The listing builds one solid part. Answer for the finished solid, in the listing's coordinates (mm). Coordinates: 2 decimals unless noted, no trailing zeros. Write each loop counter-clockwise with the first axis right and the second up, starting at its lowest first coordinate (ties: lowest second). Pieces come first, ordered by that corner, then holes. Notation, with made-up numbers: M 88.5,42 L 103.5,42 A22 ccw 103.5,54 Z; hole C -38,84 d9. An arc over 180 degrees is marked long. Answer as CSV lines item,"result". Start each with the question number.
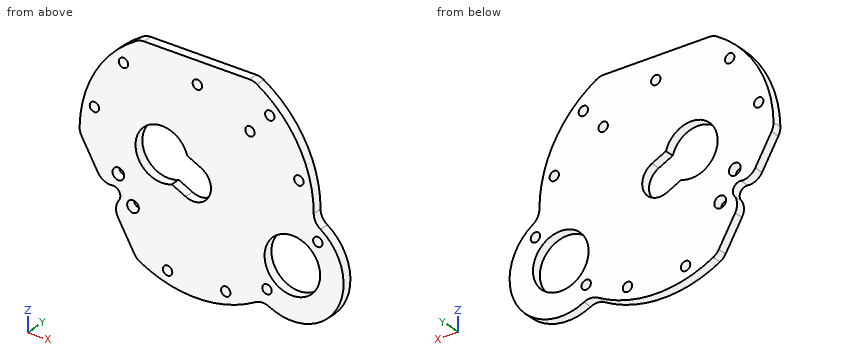
```python
from build123d import *

# Parameters (mm, degrees)
SKETCH2_R           = 9.5
SKETCH2_R_2         = 1.599999999
BOSS_EXTRUDE1_DEPTH = 3.175
FILLET1_R           = 5
CUT_EXTRUDE1_REACH  = 5.175
SKETCH3_R           = 2
FILLET2_R           = 5


with BuildPart() as part:
    # Sketch2 → Boss-Extrude1 (new body)
    with BuildSketch(Plane(origin=(0, 0, 0), x_dir=(1, 0, 0), z_dir=(0, 1, 0))):
        with BuildLine():
            Line((-20.628430767, 34.270509831), (-39.993347498, 0.729490169))
            ThreePointArc((-39.993347498, 0.729490169), (-34.641016151, -20), (-19.364916731, -35))
            Line((-19.364916731, -35), (19.364916731, -35))
            ThreePointArc((19.364916731, -35), (35.177698311, -19.040208548), (39.892817403, 2.92628085))
            ThreePointArc((39.892817403, 2.92628085), (47.858623368, 27.631189084), (22.480642256, 33.085052875))
            ThreePointArc((22.480642256, 33.085052875), (1.09954486, 39.984884658), (-20.628430767, 34.270509831))
        make_face()
        with Locations((32.703178801, 18.881189084)):
            Circle(SKETCH2_R, mode=Mode.SUBTRACT)
        with Locations((-9.933234274, 34.602468942)):
            Circle(SKETCH2_R_2, mode=Mode.SUBTRACT)
        with Locations((34.933234274, -8.698801248)):
            Circle(SKETCH2_R_2, mode=Mode.SUBTRACT)
        with Locations((24.025546071, 29.222789066)):
            Circle(SKETCH2_R_2, mode=Mode.SUBTRACT)
        with Locations((41.380811532, 8.539589102)):
            Circle(SKETCH2_R_2, mode=Mode.SUBTRACT)
        with Locations((9.933234274, 34.602468942)):
            Circle(SKETCH2_R_2, mode=Mode.SUBTRACT)
        with Locations((18.218514563, -18.662886757)):
            Circle(SKETCH2_R_2, mode=Mode.SUBTRACT)
        with Locations((-25, -25.903667694)):
            Circle(SKETCH2_R_2, mode=Mode.SUBTRACT)
        with Locations((0.242633637, -27.430309692)):
            Circle(SKETCH2_R_2, mode=Mode.SUBTRACT)
        with Locations((25, -25.903667694)):
            Circle(SKETCH2_R_2, mode=Mode.SUBTRACT)
        with Locations((-34.933234274, -8.698801248)):
            Circle(SKETCH2_R_2, mode=Mode.SUBTRACT)
        with BuildLine():
            Line((-3.733919578, 9.237483049), (-8.490154378, 6.917712338))
            ThreePointArc((-8.490154378, 6.917712338), (-19.978367669, -5.361075311), (-3.229700616, -3.867816217))
            Line((-3.229700616, -3.867816217), (1.526534184, -1.548045507))
            ThreePointArc((1.526534184, -1.548045507), (4.289071581, 6.474945652), (-3.733919578, 9.237483049))
        make_face(mode=Mode.SUBTRACT)
    extrude(amount=BOSS_EXTRUDE1_DEPTH)

    # Fillet1
    fillet1_edges = [part.edges().sort_by_distance(p)[0] for p in [
        (39.892817403, 1.5875, -2.92628085),
        (22.480642256, 1.5875, -33.085052875),
    ]]
    fillet(fillet1_edges, radius=FILLET1_R)

    # Sketch3 → Cut-Extrude1 (cut, up to next)
    with BuildSketch(Plane(origin=(0, 3.175, 0), x_dir=(1, 0, 0), z_dir=(0, 1, 0)), mode=Mode.PRIVATE) as cut_extrude1_sk1:
        with Locations((-26.748711306, 9.669872981)):
            Circle(SKETCH3_R)
    cut_extrude1_tool1 = extrude(cut_extrude1_sk1.sketch, amount=-CUT_EXTRUDE1_REACH, mode=Mode.PRIVATE) & part.part
    add(cut_extrude1_tool1.solids().sort_by_distance((-26.748711, 3.175, -9.669873))[0], mode=Mode.SUBTRACT)
    # Sketch3 → Cut-Extrude1 (cut, up to next)
    with BuildSketch(Plane(origin=(0, 3.175, 0), x_dir=(1, 0, 0), z_dir=(0, 1, 0)), mode=Mode.PRIVATE) as cut_extrude1_sk2:
        with Locations((-21.748711306, 18.330127019)):
            Circle(SKETCH3_R)
    cut_extrude1_tool2 = extrude(cut_extrude1_sk2.sketch, amount=-CUT_EXTRUDE1_REACH, mode=Mode.PRIVATE) & part.part
    add(cut_extrude1_tool2.solids().sort_by_distance((-21.748711, 3.175, -18.330127))[0], mode=Mode.SUBTRACT)
    # Sketch3 → Cut-Extrude1 (cut, up to next)
    with BuildSketch(Plane(origin=(0, 3.175, 0), x_dir=(1, 0, 0), z_dir=(0, 1, 0)), mode=Mode.PRIVATE) as cut_extrude1_sk3:
        with BuildLine():
            Line((-29.060889132, 19.665063509), (-27.328838325, 18.665063509))
            ThreePointArc((-27.328838325, 18.665063509), (-26.413774815, 15.25), (-29.828838325, 14.334936491))
            Line((-29.828838325, 14.334936491), (-31.560889132, 15.334936491))
            ThreePointArc((-31.560889132, 15.334936491), (-32.475952642, 18.75), (-29.060889132, 19.665063509))
        make_face()
    cut_extrude1_tool3 = extrude(cut_extrude1_sk3.sketch, amount=-CUT_EXTRUDE1_REACH, mode=Mode.PRIVATE) & part.part
    add(cut_extrude1_tool3.solids().sort_by_distance((-29.444864, 3.175, -17))[0], mode=Mode.SUBTRACT)

    # Fillet2
    fillet2_edges = [part.edges().sort_by_distance(p)[0] for p in [
        (-31.560889132, 1.5875, -15.334936491),
        (-29.060889132, 1.5875, -19.665063509),
        (19.364916731, 1.5875, 35),
        (-19.364916731, 1.5875, 35),
        (-39.993347498, 1.5875, -0.729490169),
        (-20.628430767, 1.5875, -34.270509831),
    ]]
    fillet(fillet2_edges, radius=FILLET2_R)


solid = part.part
```
1) The part is cut by section A-A (x = -15.5). Determine the outline of the cut face in (y, z) (3 decimals), then the cut area to 3 significant figures.
2) Find the intervals of material crossed by line 1 (X direction, y = 2.05, z = 25); line 2 (Z direction, x = -25, y = 1.25); line 3 (X direction, y = 1.3, z = -18.5), in increasing order. Write a range as from..to.
3) The part is cut by section C-C (y = 1.25). Count the separate pieces of the cut face and the enclosed holes in it, then the cut area to 3 significant figures.
4) The part is cut by section B-B (z = 21.5). Determine the outline of the cut face in (x, y) (3 decimals), then the cut area to 3 significant figures.
5) This flat-tipped pin is pushed along its axis until it touches: P1, Ø1.5, axis at y = 1, z = -3.5, coming from the -X side. Where does it stop, or does it pass through?
Completed:
1,outline,"M 0,-36.875 L 3.175,-36.875 L 3.175,-6.828 L 0,-6.828 Z; M 0,9.66 L 3.175,9.66 L 3.175,35 L 0,35 Z"
1,area,"176 mm²"
2,line 1,"-31.22..-26.32, -23.68..23.68, 26.32..31.22"
2,line 2,"-26.7..-10.64, -8.7..24.3, 27.5..31.22"
2,line 3,"-26.9..-23.74, -19.76..23.21, 42.2..50.2"
3,separate pieces,"1"
3,enclosed holes,"14"
3,area,"4,440 mm²"
4,outline,"M -33.731,0 L 33.731,0 L 33.731,3.175 L -33.731,3.175 Z"
4,area,"214 mm²"
5,P1,"x = -38.83"
